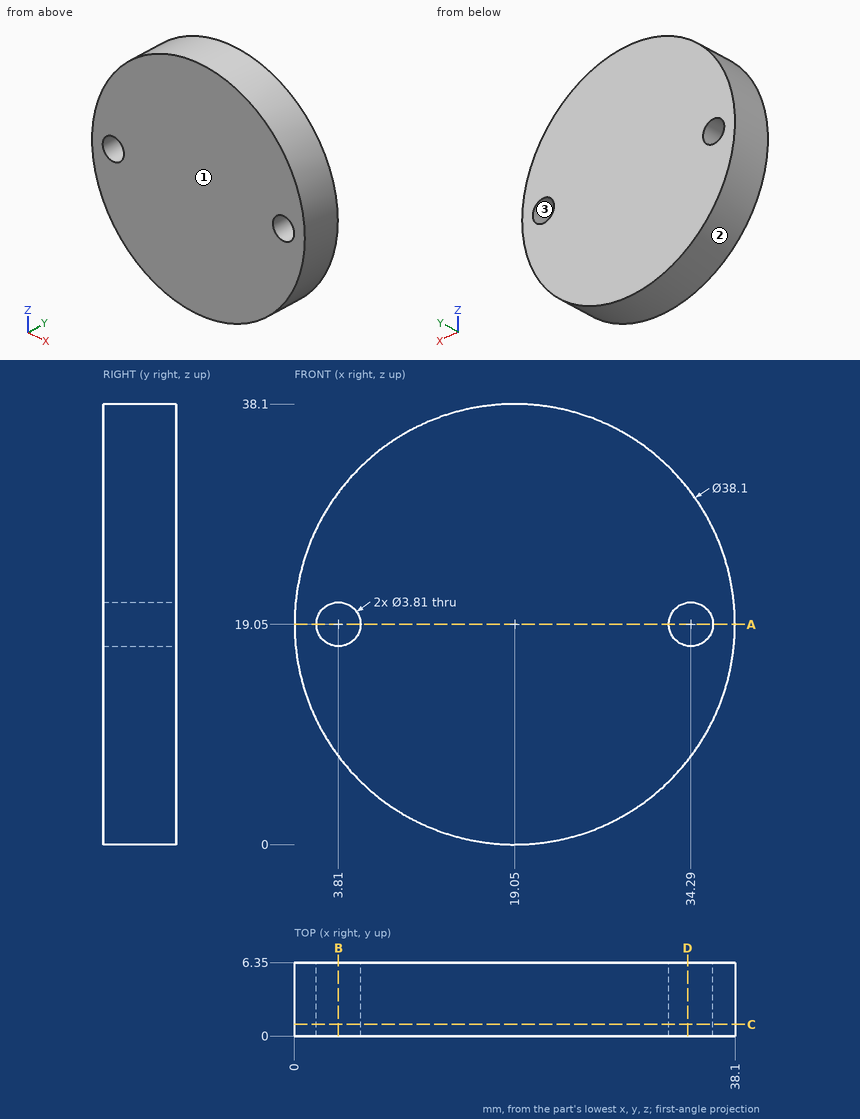
Could you check a few things on this drawing? It's one solid part, dimensions in mm from its lowest x, y, z. Round coordinates to 2 decimals unless told otherwise and drop trailing zeros. Loops run counter-clockwise (first coordinate to the right, second up) from the corner with the lowest first, then second, coordinate; pieces in that order, holes last. Notation, with made-up numbers: M -37.5,4 L 16.5,4 A27 cw 16.5,39 Z; hole C 84.5,-37.5 d3. An arc over 180 degrees is marked long. Write each question's results on one line, items separated by ' | '. Start each with the question number.
(1) I want a section at D-D (x = 34). Please give me the cut outline in (y, z), then the cut area to 3 significant figures.
(2) I want a section at B-B (x = 3.81). Please give me the cut outline in (y, z) (3 decimals), then the cut area to 3 significant figures.
(3) I want a section at A-A (z = 19.05). Please give me the cut outline in (x, y) (3 decimals), then the cut area to 3 significant figures.
(4) If I drill on probe 1 along Z at (x, y) = (35, 1.75); probe 2 along Z at (x, y) = (18.5, 1); probe 3 along Z at (x, y) = (4, 2.25), over which ranges is the centre line in solid material (lowest first)? Write a range as from..to.
(5) Will this pin go through, and if not, where does the flat tip stop? P1, Ø2.5, axis at x = 3.81, z = 19.05, coming from the +Y side.
(6) Thinking about a two-plate mould opening in X: for the marked faces 1, 2 and 3, which applies, pulls with the +X half, pulls with the -X half, needs draft (parallel to the pull), parting line crosses it, or undercut?
(7) I want a section at C-C (y = 1). Please give me the cut outline in (x, z) (3 decimals).
Solved:
1) outline: M 0,7.24 L 6.35,7.24 L 6.35,17.17 L 0,17.17 Z; M 0,20.93 L 6.35,20.93 L 6.35,30.86 L 0,30.86 Z | area: 126 mm²
2) outline: M 0,7.62 L 6.35,7.62 L 6.35,17.145 L 0,17.145 Z; M 0,20.955 L 6.35,20.955 L 6.35,30.48 L 0,30.48 Z | area: 121 mm²
3) outline: M 0,0 L 1.905,0 L 1.905,6.35 L 0,6.35 Z; M 5.715,0 L 32.385,0 L 32.385,6.35 L 5.715,6.35 Z; M 36.195,0 L 38.1,0 L 38.1,6.35 L 36.195,6.35 Z | area: 194 mm²
4) probe 1: z = 8.63..17.28, 20.82..29.47 | probe 2: z = 0.01..38.09 | probe 3: z = 7.37..17.15, 20.95..30.73
5) P1: passes through
6) face 1: needs draft | face 2: parting line crosses it | face 3: undercut
7) outline: C 19.05,19.05 d38.1; hole C 3.81,19.05 d3.81; hole C 34.29,19.05 d3.81
